Part model, mm, in its own coordinate system. A direction names the side the tool comes from. Give positions to 0.01 mm unless a question says otherwise; leave off trailing zeros. Write each loop counter-clockwise with the first axis right and the second up, starting at its lowest first coordinate (ties: lowest second). Pieces come first, ordered by that corner, then holes. Notation, with made-up numbers: M 53,78 L 73,78 A20 cw 73,85 Z; hole C 36.5,-38 d9. An arc over 180 degrees is marked long. Use a Markdown table: item, result. Add a question column.
from build123d import *

# Parameters (mm, degrees)
F0_R      = 9.5
F1_DEPTH  = 28
F3_DEPTH  = 6
F5_R      = 6
F6_DEPTH  = 22.001
F7_W      = 13
F7_H      = 63.7986809015
F8_DEPTH  = 38
F10_DEPTH = 6


with BuildPart() as f1:
    # F0 (on Front) → F1 (new body)
    with BuildSketch(Plane.XZ):
        with BuildLine():
            Line((55.3299104147, -19.4800459675), (55.27629582, -7.5791569764))
            ThreePointArc((55.27629582, -7.5791569764), (21.8781261357, 2.6281537564), (-1.8464281096, 28.2557259496))
            ThreePointArc((-1.8464281096, 28.2557259496), (-18.2536420422, 35.1646349887), (-28.1767553192, 20.3841912865))
            Line((-28.1767553192, 20.3841912865), (-23.4563932978, -27.7273269018))
            ThreePointArc((-23.4563932978, -27.7273269018), (-15.7507812014, -42.3917991939), (0, -47.5236698985))
            Line((0, -47.5236698985), (55.4384774708, -43.5787916566))
            Line((55.4384774708, -43.5787916566), (55.3839715136, -31.4800459675))
            Line((55.3839715136, -31.4800459675), (33.3841947645, -31.5791569764))
            ThreePointArc((33.3841947645, -31.5791569764), (27.3571642151, -25.6061875258), (33.3301336657, -19.5791569764))
            Line((33.3301336657, -19.5791569764), (55.3299104147, -19.4800459675))
        make_face()
        with Locations((-1.5615225292, -25.5791569764)):
            Circle(F0_R, mode=Mode.SUBTRACT)
    extrude(amount=F1_DEPTH)

    # F2 (on face) → F3 (cut)
    with BuildSketch(Plane.XZ.offset(28)):
        with BuildLine():
            ThreePointArc((4.462620132, 18.4232597398), (4.6827707797, 20.0807656893), (4.7563442608, 21.7512085118))
            ThreePointArc((4.7563442608, 21.7512085118), (-21.9929159378, 39.0990892578), (-26.9224943051, 7.6003409546))
            Line((-26.9224943051, 7.6003409546), (-28.1767553192, 20.3841912865))
            ThreePointArc((-28.1767553192, 20.3841912865), (-18.2536420422, 35.1646349887), (-1.8464281096, 28.2557259496))
            ThreePointArc((-1.8464281096, 28.2557259496), (1.0933811252, 23.2017200271), (4.462620132, 18.4232597398))
        make_face()
        with BuildLine():
            ThreePointArc((6.5586960689, 15.8448641244), (5.4946710371, 17.1210654398), (4.462620132, 18.4232597398))
            ThreePointArc((4.462620132, 18.4232597398), (4.1823746256, 17.1164048487), (3.8109479717, 15.8324852676))
            Line((3.8109479717, 15.8324852676), (6.5586960689, 15.8448641244))
        make_face()
        with BuildLine():
            Line((-28.1767553192, 20.3841912865), (-26.9224943051, 7.6003409546))
            ThreePointArc((-26.9224943051, 7.6003409546), (-9.3276855683, 3.3981913953), (3.8109479717, 15.8324852676))
            ThreePointArc((3.8109479717, 15.8324852676), (4.1823746256, 17.1164048487), (4.462620132, 18.4232597398))
            ThreePointArc((4.462620132, 18.4232597398), (1.0933811252, 23.2017200271), (-1.8464281096, 28.2557259496))
            ThreePointArc((-1.8464281096, 28.2557259496), (-18.2536420422, 35.1646349887), (-28.1767553192, 20.3841912865))
        make_face()
    extrude(amount=-F3_DEPTH, mode=Mode.SUBTRACT)

    # F5 (on face) → F6 (cut, through all)
    with BuildSketch(Plane.XZ.offset(22)):
        with Locations((-14.2436557392, 21.7512085118)):
            Circle(F5_R)
    extrude(amount=-F6_DEPTH, mode=Mode.SUBTRACT)

    # F7 (on face) → F8 (cut)
    with BuildSketch(Plane(origin=(55.2410298601, 0, 0.248865898), x_dir=(0, 1, 0), z_dir=(0.9999898522, 0, 0.0045050459))):
        with Locations((-14, -22.6326100528)):
            Rectangle(F7_W, F7_H)
    extrude(amount=-F8_DEPTH, mode=Mode.SUBTRACT)

    # F9 (on face) → F10 (cut)
    with BuildSketch(Plane(origin=(0, 0, 0), x_dir=(-1, 0, 0), z_dir=(0, 1, 0))):
        with BuildLine():
            ThreePointArc((-3.7841006381, 15.7512085118), (17.2827862753, 2.9958443302), (33.2436557392, 21.7512085118))
            ThreePointArc((33.2436557392, 21.7512085118), (11.2045252031, 40.5065726934), (-3.7841006381, 15.7512085118))
        make_face()
        with BuildLine():
            ThreePointArc((-3.7841006381, 15.7512085118), (-4.1718878517, 17.0749114458), (-4.462620132, 18.4232597398))
            ThreePointArc((-4.462620132, 18.4232597398), (-5.5335871793, 17.0732394365), (-6.6389194686, 15.7512085118))
            Line((-6.6389194686, 15.7512085118), (-3.7841006381, 15.7512085118))
        make_face()
    extrude(amount=-F10_DEPTH, mode=Mode.SUBTRACT)


solid = f1.part
1. Cut at C-C (z = 26). Write the cut outline in (x, y).
2. Tool access for faces 1 (the flat face through (-25.85, -13.8, -3.33)), 2 (the flat face through (5, -3, 15.751)): list every direction of +Z, -Z, +X, -X, +Y, -Y with a clear straight run to the whole face (end or side of a thin tool).
3. Flat gauge pins, fed straight in: pin 1 (12 mm diameter, centred on x = 5, y = -10.5, fed in from -Z); pin 2 (2 mm diameter, centred on y = -13.5, z = 1.5, fed in from +X); pin 3 (1.5 mm diameter, centred on x = -8, y = -23.5, fed in from -Z); pin 4 (10 mm diameter, centred on x = -2.5, z = 12.5, fed in from -Y). Where does each tip first touch, or does it go through?
4. Cut at A-A (x = -14.5). Write the cut outline in (y, z), then the cut area to 3 significant figures.
5. Cut at B-B (y = -2.25). Write the cut outline in (x, z).
6. Drill centre lines: probe 1 along Y at (x, z) = (44.5, -18.5); probe 2 along Z at (x, y) = (0, -5); probe 3 along X at (y, z) = (-10, -23.5). Where is each one in solid material? Low to high. Write a range as [from, to].
7. Cut at D-D (y = -12.5). Write the cut outline in (x, z).
8. Mould opens along X. For faces 3 (the flat face through (14, -28, -22)), 4 (the cylindrical face through (-11.475, -14.112, 16.428)), 5 (the flat face through (15.012, -13.804, -46.455)) say: released by +X, released by -X, zero draft, split by the parting line, or undercut.
A:
| question | item | result |
|---|---|---|
| 1 | outline | M -27.58,-22 L -18.48,-22 L -18.48,-6 L -27.58,-6 Z; M -10.01,-22 L -0.61,-22 L -0.61,-6 L -10.01,-6 Z |
| 2 | face 1 | -Z, -X, +Y, -Y |
| 2 | face 2 | +Z, +X, -X, +Y |
| 3 | pin 1 | stops at z = -47.57 |
| 3 | pin 2 | stops at x = 17.24 |
| 3 | pin 3 | stops at z = -46.83 |
| 3 | pin 4 | stops at y = -28 |
| 4 | outline | M -28,-43.37 L 0,-43.37 L 0,2.75 L -6,2.75 L -6,15.76 L -22,15.76 L -22,2.75 L -28,2.75 Z; M -22,27.75 L -6,27.75 L -6,35.75 L -22,35.75 Z |
| 4 | area | 1,630 mm² |
| 5 | outline | M -26.92,7.6 L -23.46,-27.73 A22 ccw 0,-47.52 L 55.44,-43.58 L 55.38,-31.48 L 33.38,-31.58 A6 cw 33.33,-19.58 L 55.33,-19.48 L 55.28,-7.58 A67 cw 6.64,15.75 L 3.78,15.75 A19 cw Z; hole C -1.56,-25.58 d19 |
| 6 | probe 1 | y = [-28, -20.5], [-7.5, 0] |
| 6 | probe 2 | z = [-47.52, -34.95], [-16.21, 9.18] |
| 6 | probe 3 | x = [-23.87, -10.83], [7.71, 17.35] |
| 7 | outline | M -28.18,20.38 L -23.46,-27.73 A22 ccw 0,-47.52 L 17.45,-46.28 L 17.22,5.84 A67 cw -1.85,28.26 A14 ccw Z; hole C -14.24,21.75 d12; hole C -1.56,-25.58 d19 |
| 8 | face 3 | zero draft |
| 8 | face 4 | undercut |
| 8 | face 5 | released by +X |
